```python
from build123d import *

# Parameters (mm, degrees)
CYLINDER077_R             = 1.25
CYLINDER077_DEPTH         = 15
CYLINDER078_R             = 1.25
CYLINDER078_DEPTH         = 15
CYLINDER081_R             = 1.25
CYLINDER081_DEPTH         = 15
CYLINDER082_R             = 1.25
CYLINDER082_DEPTH         = 15
FUSION041_PLACEMENT_ANGLE = 90
CYLINDER079_R             = 11
CYLINDER079_DEPTH         = 4.5
CYLINDER080_R             = 2.6
CYLINDER080_DEPTH         = 12
BOX006_W                  = 26
BOX006_H                  = 26
BOX006_DEPTH              = 12
CUT014015_PLACEMENT_ANGLE = 180


with BuildPart() as cylinder077:
    # Cylinder077 → Cylinder077 (new body)
    with BuildSketch(Plane(origin=(7, 0, 0), x_dir=(1, 0, 0), z_dir=(0, 0, 1))):
        Circle(CYLINDER077_R)
    extrude(amount=CYLINDER077_DEPTH)


with BuildPart() as fusion042:
    # Cylinder078 → Cylinder078 (new body)
    with BuildSketch(Plane(origin=(-7, 0, 0), x_dir=(1, 0, 0), z_dir=(0, 0, 1))):
        Circle(CYLINDER078_R)
    extrude(amount=CYLINDER078_DEPTH)

    # Fusion042: union Cylinder077
    add(cylinder077.part)


with BuildPart() as cylinder081:
    # Cylinder081 → Cylinder081 (new body)
    with BuildSketch(Plane(origin=(7, 0, 0), x_dir=(1, 0, 0), z_dir=(0, 0, 1))):
        Circle(CYLINDER081_R)
    extrude(amount=CYLINDER081_DEPTH)


with BuildPart() as fusion043:
    # Cylinder082 → Cylinder082 (new body)
    with BuildSketch(Plane(origin=(-7, 0, 0), x_dir=(1, 0, 0), z_dir=(0, 0, 1))):
        Circle(CYLINDER082_R)
    extrude(amount=CYLINDER082_DEPTH)

    # Fusion041: union Cylinder081
    add(cylinder081.part)


with BuildPart() as fusion043_1:
    # Fusion041 placement: moved
    add(fusion043.part.rotate(Axis((0, 0, 0), (0, 0, 1)), FUSION041_PLACEMENT_ANGLE))

    # Fusion043: union Fusion042
    add(fusion042.part)


with BuildPart() as fusion043_2:
    # Fusion043 placement: moved
    add(fusion043_1.part.moved(Location((0, 0, -3))))


with BuildPart() as cylinder079:
    # Cylinder079 → Cylinder079 (new body)
    with BuildSketch(Plane.XY):
        Circle(CYLINDER079_R)
    extrude(amount=CYLINDER079_DEPTH)


with BuildPart() as fusion040:
    # Cylinder080 → Cylinder080 (new body)
    with BuildSketch(Plane.XY):
        Circle(CYLINDER080_R)
    extrude(amount=CYLINDER080_DEPTH)

    # Fusion040: union Cylinder079
    add(cylinder079.part)


with BuildPart() as diff_lock_holes:
    # Box006 → Box006 (new body)
    with BuildSketch(Plane(origin=(-13, -13, 0), x_dir=(1, 0, 0), z_dir=(0, 0, 1))):
        with Locations((13, 13)):
            Rectangle(BOX006_W, BOX006_H)
    extrude(amount=BOX006_DEPTH)

    # Cut014014: cut Fusion040
    add(fusion040.part, mode=Mode.SUBTRACT)

    # Cut014015: cut Fusion043
    add(fusion043_2.part, mode=Mode.SUBTRACT)


with BuildPart() as diff_lock_holes_1:
    # Cut014015 placement: moved
    add(diff_lock_holes.part.moved(Location((0, 0, 31))).rotate(Axis((0, 0, 31), (0, 1, 0)), CUT014015_PLACEMENT_ANGLE))


solid = diff_lock_holes_1.part
```
Work out the finished part from the listing and answer in its coordinate system (mm). A direction names the side the tool comes from. Coordinates: 2 decimals unless noted, no trailing zeros. Loops run counter-clockwise (first coordinate to the right, second up) from the corner with the lowest first, then second, coordinate; pieces in that order, holes last. Notation, with made-up numbers: (55.25, 60) - (79.25, 60) arc R25 cw to (79.25, 84) - close; hole circle Ø1 at (27, -33). An arc over 180 degrees is marked (long way). Use a Markdown table: item, result.
Item 1: Find section C-C, the plane z = 24.5. Determine the outline of the cut face in (x, y), and give its area (3 significant figures).
Evaluation:
| item | result |
|---|---|
| outline | (-13, -13) - (13, -13) - (13, 13) - (-13, 13) - close; hole circle Ø2.5 at (-7, 0); hole circle Ø5.2 at (0, 0); hole circle Ø2.5 at (0, -7); hole circle Ø2.5 at (0, 7); hole circle Ø2.5 at (7, 0) |
| area | 635 mm2 |
Item 2: Find section A-A, the plane x = 0. Determine the outline of the cut face in (y, z).
Evaluation:
| item | result |
|---|---|
| outline | (-13, 19) - (-8.25, 19) - (-8.25, 26.5) - (-11, 26.5) - (-11, 31) - (-13, 31) - close; (-5.75, 19) - (-2.6, 19) - (-2.6, 26.5) - (-5.75, 26.5) - close; (2.6, 19) - (5.75, 19) - (5.75, 26.5) - (2.6, 26.5) - close; (8.25, 19) - (13, 19) - (13, 31) - (11, 31) - (11, 26.5) - (8.25, 26.5) - close |
Item 3: The mould has two halves that part along Y. Classify faces 3 (the flat face through (0, 3, 26.5)), 4 (the flat face through (0, -3, 19)), 5 (the flat face through (0, -13, 25)): +Y half, -Y half, draft (parallel to the pull), parting line (faces both ways), or undercut.
Evaluation:
| item | result |
|---|---|
| face 3 | undercut |
| face 4 | draft |
| face 5 | -Y half |
Item 4: Find section D-D, the plane y = 7. Determine the outline of the cut face in (x, z).
Evaluation:
| item | result |
|---|---|
| outline | (-13, 19) - (-1.25, 19) - (-1.25, 26.5) - (-8.49, 26.5) - (-8.49, 31) - (-13, 31) - close; (1.25, 19) - (13, 19) - (13, 31) - (8.49, 31) - (8.49, 26.5) - (1.25, 26.5) - close |
Item 5: Consider probe 1 along X at (y, z) = (0, 21.5); probe 2 along X at (y, z) = (7, 23); probe 3 along Y at (x, z) = (1, 24.25). Determine where each line is inside the solid, lowest interval first. Write a range as from..to.
Evaluation:
| item | result |
|---|---|
| probe 1 | x = -13..-8.25, -5.75..-2.6, 2.6..5.75, 8.25..13 |
| probe 2 | x = -13..-1.25, 1.25..13 |
| probe 3 | y = -13..-7.75, -6.25..-2.4, 2.4..6.25, 7.75..13 |
Item 6: For faces 1 (the cylindrical face through (2.38, -10.74, 28.78)), 2 (the cylindrical face through (8.25, 0.05, 22.8)), determine the directions among +Z, -Z, +X, -X, +Y, -Y from which every point of the face is accessible in a straight line to the end or side of a thin tool.
Evaluation:
| item | result |
|---|---|
| face 1 | +Z |
| face 2 | +Z, -Z |
